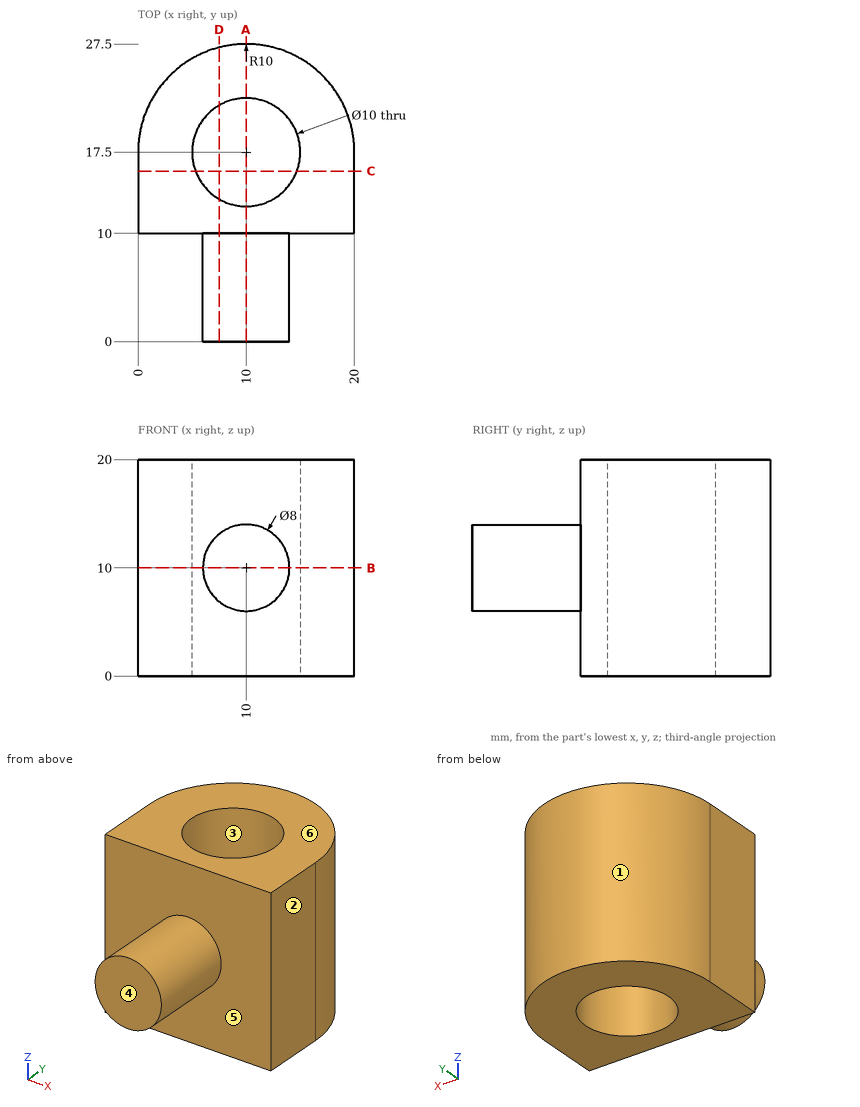
Geometry check sheet. Reference: drawing and pictorial views, mm from the part's lowest x, y, z. A direction names the side the tool comes from. Give positions to 0.01 mm unless a question says otherwise; leave off trailing zeros. Write each loop counter-clockwise with the first axis right and the second up, starting at its lowest first coordinate (ties: lowest second). Pieces come first, ordered by that corner, then holes. Notation, with made-up numbers: M 86,-30 L 138,-30 A29 cw 138,9 Z; hole C -15,-5 d1. An arc over 180 degrees is marked long. Answer as CSV lines item,"result". Start each with the question number.
Q1. Section check D-D, the plane x = 7.5. Record the cut outline in (y, z).
Q2. Release check for a two-part mould opening along Y. For the marked faces 1, 2, 3 and 4 record: pulls with the +Y half, pulls with the -Y half, needs draft (parallel to the pull), parting line crosses it, or undercut.
Q3. Section check B-B, the plane z = 10. Record the cut outline in (x, y), then the cut area to 3 significant figures.
Q4. Tool access check on the marked faces 5 and 6. Record the directions out of +Z, -Z, +X, -X, +Y, -Y that give a thin tool (end or side, any length) a straight path to the whole face; none if there is none.
Q5. Section check A-A, the plane x = 10. Record the cut outline in (y, z), then the cut area to 3 significant figures.
Q6. Section check C-C, the plane y = 15.75. Record the cut outline in (x, z).
Q7. Material ranges on L1, parallel to Y at x = 10, z = 15.5; L2, parallel to X at y = 17.25, z = 8.5; L3, parallel to Y at x = 10, z = 12, recorded low to high.
Q8. Go/stop test with flat-tipped pins: pin 1 (1.5 mm diameter, centred on y = 24, z = 8, fed in from -X); pin 2 (5 mm diameter, centred on y = 6.5, z = 14, fed in from +X); pin 3 (1.5 mm diameter, centred on y = 7, z = 9, fed in from -X). Record where each tip stops, or that it passes through.
Geometry says:
1,outline,"M 0,6.88 L 10,6.88 L 10,0 L 13.17,0 L 13.17,20 L 10,20 L 10,13.12 L 0,13.12 Z; M 21.83,0 L 27.18,0 L 27.18,20 L 21.83,20 Z"
2,face 1,"pulls with the +Y half"
2,face 2,"needs draft"
2,face 3,"undercut"
2,face 4,"pulls with the -Y half"
3,outline,"M 0,10 L 6,10 L 6,0 L 14,0 L 14,10 L 20,10 L 20,17.5 A10 ccw 0,17.5 Z; hole C 10,17.5 d10"
3,area,"309 mm^2"
4,face 5,"-Y"
4,face 6,"+Z, +X, -X, +Y, -Y"
5,outline,"M 0,6 L 10,6 L 10,0 L 12.5,0 L 12.5,20 L 10,20 L 10,14 L 0,14 Z; M 22.5,0 L 27.5,0 L 27.5,20 L 22.5,20 Z"
5,area,"230 mm^2"
6,outline,"M 0,0 L 5.32,0 L 5.32,20 L 0,20 Z; M 14.68,0 L 20,0 L 20,20 L 14.68,20 Z"
7,L1,"10 to 12.5, 22.5 to 27.5"
7,L2,"0 to 5.01, 14.99 to 20"
7,L3,"0 to 12.5, 22.5 to 27.5"
8,pin 1,"x = 1.82"
8,pin 2,"x = 13.71"
8,pin 3,"x = 6.01"
